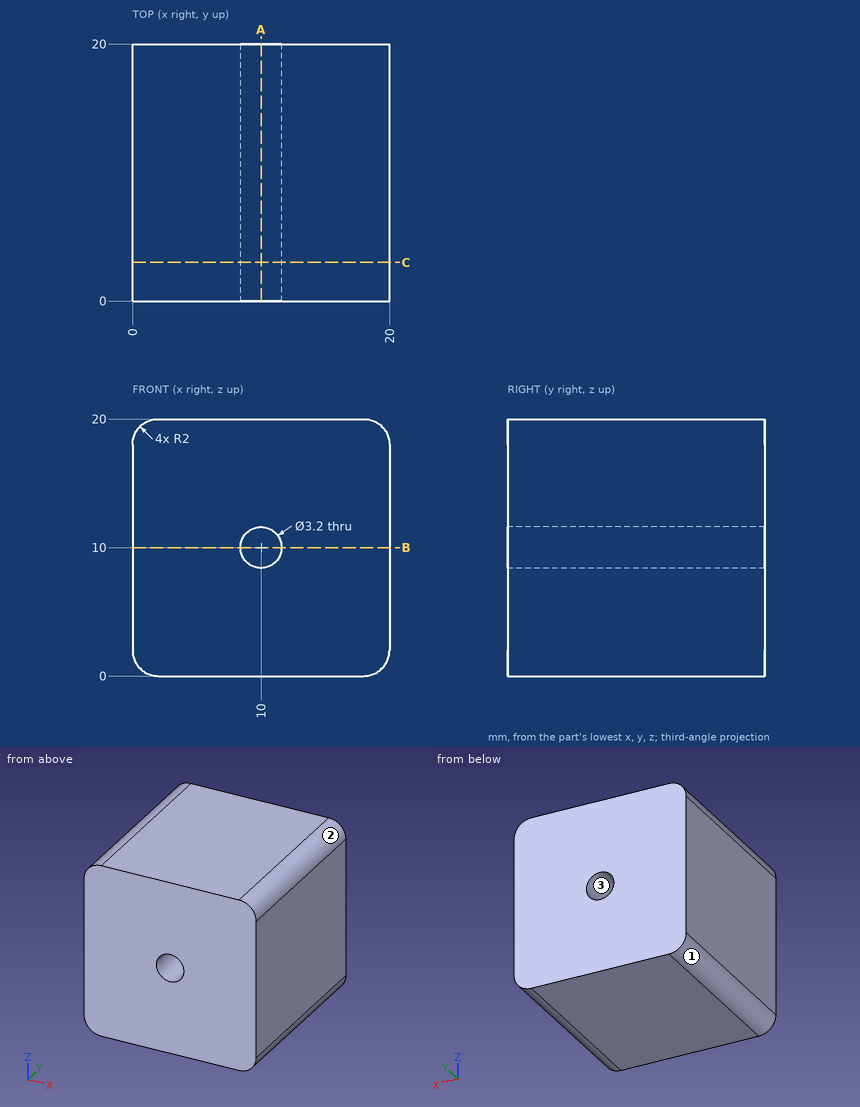
Verification items for this drawing (mm, ordinates from the low corner). Coordinates: 2 decimals unless noted, no trailing zeros. Loops run counter-clockwise (first coordinate to the right, second up) from the corner with the lowest first, then second, coordinate; pieces in that order, holes last.
Item 1: Sectioned sample at A-A, the plane x = 10. Record the boundary of the cut face in (y, z), then the cut area to 3 significant figures.
Item 2: Sectioned sample at C-C, the plane y = 3. Record the boundary of the cut face in (x, z), then the cut area to 3 significant figures.
Item 3: Release check for a two-part mould opening along Z. For the marked faces 1, 2 and 3 record: released by +Z, released by -Z, zero draft, split by the parting line, or undercut.
Item 4: Sectioned sample at B-B, the plane z = 10. Record the boundary of the cut face in (x, y).
Item 5: Go/stop test with a flat-tipped pin: pin 1 Ø2.5 at (x, z) = (10, 10) entering from +Y. Record where the tip stops, or that it passes through.
Item 6: Thickness scan on line 1 (X direction, y = 17, z = 10); line 2 (X direction, y = 5.5, z = 9.5). Record the ranges inside material, lowest first.
Check result:
1. outline: (0, 0) - (20, 0) - (20, 8.4) - (0, 8.4) - close; (0, 11.6) - (20, 11.6) - (20, 20) - (0, 20) - close
1. area: 336 mm2
2. outline: (0, 2) arc R2 ccw to (2, 0) - (18, 0) arc R2 ccw to (20, 2) - (20, 18) arc R2 ccw to (18, 20) - (2, 20) arc R2 ccw to (0, 18) - close; hole circle Ø3.2 at (10, 10)
2. area: 389 mm2
3. face 1: released by -Z
3. face 2: released by +Z
3. face 3: undercut
4. outline: (0, 0) - (8.4, 0) - (8.4, 20) - (0, 20) - close; (11.6, 0) - (20, 0) - (20, 20) - (11.6, 20) - close
5. pin 1: passes through
6. line 1: x = 0 to 8.4, 11.6 to 20
6. line 2: x = 0 to 8.48, 11.52 to 20
